from build123d import *

# Parameters (mm, degrees)
F0_R     = 2.5527
F0_R_2   = 14.2875
F0_W     = 25.4
F0_H     = 50.8
F1_DEPTH = 6


with BuildPart() as f1:
    # F0 (on Right) → F1 (new body)
    with BuildSketch(Plane.YZ):
        Polygon((177.8, 139.7), (0, 25.4), (0, -25.4), (177.8, -25.4), (177.8, -139.7), (444.5, -139.7), (444.5, 139.7), align=None)
        with Locations((190.5, -127)):
            Circle(F0_R, mode=Mode.SUBTRACT)
        with Locations((215.9, -127)):
            Circle(F0_R, mode=Mode.SUBTRACT)
        with Locations((190.5, -101.6)):
            Circle(F0_R, mode=Mode.SUBTRACT)
        with Locations((215.9, -101.6)):
            Circle(F0_R, mode=Mode.SUBTRACT)
        with Locations((190.5, -76.2)):
            Circle(F0_R, mode=Mode.SUBTRACT)
        with Locations((215.9, -76.2)):
            Circle(F0_R, mode=Mode.SUBTRACT)
        with Locations((4.77777, -11.90625)):
            Circle(F0_R, mode=Mode.SUBTRACT)
        with Locations((46.02223, -11.90625)):
            Circle(F0_R, mode=Mode.SUBTRACT)
        with Locations((63.5, -12.7)):
            Circle(F0_R, mode=Mode.SUBTRACT)
        with Locations((88.9, -12.7)):
            Circle(F0_R, mode=Mode.SUBTRACT)
        with Locations((190.5, -50.8)):
            Circle(F0_R, mode=Mode.SUBTRACT)
        with Locations((215.9, -50.8)):
            Circle(F0_R, mode=Mode.SUBTRACT)
        with Locations((114.3, -12.7)):
            Circle(F0_R, mode=Mode.SUBTRACT)
        with Locations((139.7, -12.7)):
            Circle(F0_R, mode=Mode.SUBTRACT)
        with Locations((165.1, -12.7)):
            Circle(F0_R, mode=Mode.SUBTRACT)
        with Locations((190.5, -25.4)):
            Circle(F0_R, mode=Mode.SUBTRACT)
        with Locations((215.9, -25.4)):
            Circle(F0_R, mode=Mode.SUBTRACT)
        with Locations((190.5, -12.7)):
            Circle(F0_R, mode=Mode.SUBTRACT)
        with Locations((215.9, -12.7)):
            Circle(F0_R, mode=Mode.SUBTRACT)
        with Locations((241.3, -127)):
            Circle(F0_R, mode=Mode.SUBTRACT)
        with Locations((266.7, -127)):
            Circle(F0_R, mode=Mode.SUBTRACT)
        with Locations((292.1, -127)):
            Circle(F0_R, mode=Mode.SUBTRACT)
        with Locations((317.5, -127)):
            Circle(F0_R, mode=Mode.SUBTRACT)
        with Locations((241.3, -101.6)):
            Circle(F0_R, mode=Mode.SUBTRACT)
        with Locations((266.7, -101.6)):
            Circle(F0_R, mode=Mode.SUBTRACT)
        with Locations((292.1, -101.6)):
            Circle(F0_R, mode=Mode.SUBTRACT)
        with Locations((317.5, -101.6)):
            Circle(F0_R, mode=Mode.SUBTRACT)
        with Locations((342.9, -127)):
            Circle(F0_R, mode=Mode.SUBTRACT)
        with Locations((368.3, -127)):
            Circle(F0_R, mode=Mode.SUBTRACT)
        with Locations((393.7, -127)):
            Circle(F0_R, mode=Mode.SUBTRACT)
        with Locations((419.1, -127)):
            Circle(F0_R, mode=Mode.SUBTRACT)
        with Locations((342.9, -101.6)):
            Circle(F0_R, mode=Mode.SUBTRACT)
        with Locations((368.3, -101.6)):
            Circle(F0_R, mode=Mode.SUBTRACT)
        with Locations((393.7, -101.6)):
            Circle(F0_R, mode=Mode.SUBTRACT)
        with Locations((419.1, -101.6)):
            Circle(F0_R, mode=Mode.SUBTRACT)
        with Locations((25.4, 0)):
            Circle(F0_R_2, mode=Mode.SUBTRACT)
        with Locations((4.77777, 11.90625)):
            Circle(F0_R, mode=Mode.SUBTRACT)
        with Locations((46.02223, 11.90625)):
            Circle(F0_R, mode=Mode.SUBTRACT)
        with Locations((63.5, 12.7)):
            Circle(F0_R, mode=Mode.SUBTRACT)
        with Locations((88.9, 12.7)):
            Circle(F0_R, mode=Mode.SUBTRACT)
        with Locations((114.3, 12.7)):
            Circle(F0_R, mode=Mode.SUBTRACT)
        with Locations((139.7, 12.7)):
            Circle(F0_R, mode=Mode.SUBTRACT)
        with Locations((165.1, 12.7)):
            Circle(F0_R, mode=Mode.SUBTRACT)
        with Locations((190.5, 0)):
            Circle(F0_R, mode=Mode.SUBTRACT)
        with Locations((190.5, 12.7)):
            Circle(F0_R, mode=Mode.SUBTRACT)
        with Locations((215.9, 0)):
            Circle(F0_R, mode=Mode.SUBTRACT)
        with Locations((215.9, 12.7)):
            Circle(F0_R, mode=Mode.SUBTRACT)
        with Locations((190.5, 25.4)):
            Circle(F0_R, mode=Mode.SUBTRACT)
        with Locations((215.9, 25.4)):
            Circle(F0_R, mode=Mode.SUBTRACT)
        with Locations((165.1, 50.8)):
            Rectangle(F0_W, F0_H, mode=Mode.SUBTRACT)
        with Locations((190.5, 50.8)):
            Circle(F0_R, mode=Mode.SUBTRACT)
        with Locations((215.9, 50.8)):
            Circle(F0_R, mode=Mode.SUBTRACT)
        with Locations((190.5, 76.2)):
            Circle(F0_R, mode=Mode.SUBTRACT)
        with Locations((215.9, 76.2)):
            Circle(F0_R, mode=Mode.SUBTRACT)
        with Locations((190.5, 101.6)):
            Circle(F0_R, mode=Mode.SUBTRACT)
        with Locations((215.9, 101.6)):
            Circle(F0_R, mode=Mode.SUBTRACT)
        with Locations((190.5, 127)):
            Circle(F0_R, mode=Mode.SUBTRACT)
        with Locations((215.9, 127)):
            Circle(F0_R, mode=Mode.SUBTRACT)
        with Locations((241.3, 101.6)):
            Circle(F0_R, mode=Mode.SUBTRACT)
        with Locations((266.7, 101.6)):
            Circle(F0_R, mode=Mode.SUBTRACT)
        with Locations((292.1, 101.6)):
            Circle(F0_R, mode=Mode.SUBTRACT)
        with Locations((317.5, 101.6)):
            Circle(F0_R, mode=Mode.SUBTRACT)
        with Locations((241.3, 127)):
            Circle(F0_R, mode=Mode.SUBTRACT)
        with Locations((266.7, 127)):
            Circle(F0_R, mode=Mode.SUBTRACT)
        with Locations((292.1, 127)):
            Circle(F0_R, mode=Mode.SUBTRACT)
        with Locations((317.5, 127)):
            Circle(F0_R, mode=Mode.SUBTRACT)
        with Locations((342.9, 101.6)):
            Circle(F0_R, mode=Mode.SUBTRACT)
        with Locations((368.3, 101.6)):
            Circle(F0_R, mode=Mode.SUBTRACT)
        with Locations((393.7, 101.6)):
            Circle(F0_R, mode=Mode.SUBTRACT)
        with Locations((342.9, 127)):
            Circle(F0_R, mode=Mode.SUBTRACT)
        with Locations((368.3, 127)):
            Circle(F0_R, mode=Mode.SUBTRACT)
        with Locations((419.1, 114.3)):
            Circle(F0_R_2, mode=Mode.SUBTRACT)
        with Locations((393.7, 127)):
            Circle(F0_R, mode=Mode.SUBTRACT)
    extrude(amount=F1_DEPTH)


solid = f1.part
Check sheet for the modelled part. Datum: model origin and axes. Units: mm. Give positions to 0.01 mm unless a question says otherwise; leave off trailing zeros. Write each loop counter-clockwise with the first axis right and the second up, starting at its lowest first coordinate (ties: lowest second). Pieces come first, ordered by that corner, then holes. Notation, with made-up numbers: (-21, 50) -> (-17, 50) arc R32 cw to (-17, 88) -> close; hole circle Ø9 at (13.25, -38). An arc over 180 degrees is marked (long way). Write item = value, one per line.
Item 1: Sectioned sample at B-B on z = -38. Record the boundary of the cut face in (x, y), and give its area (3 significant figures).
Output:
outline = (0, 177.8) -> (6, 177.8) -> (6, 444.5) -> (0, 444.5) -> close
area = 1,600 mm^2
Item 2: Sectioned sample at C-C on x = 1. Count the separate pieces of the cut face and the enclosed holes in it, and give its area (3 significant figures).
Output:
separate_pieces = 1
enclosed_holes = 73
area = 89,700 mm^2
Item 3: Sectioned sample at A-A on y = 25.4. Record the boundary of the cut face in (x, z).
Output:
outline = (0, -25.4) -> (6, -25.4) -> (6, -14.29) -> (0, -14.29) -> close; (0, 14.29) -> (6, 14.29) -> (6, 41.73) -> (0, 41.73) -> close
Item 4: Scan lines: probe 1 along Z at (x, y) = (1, 292); probe 2 along Y at (x, z) = (4.45, 2); probe 3 along Z at (x, y) = (2.45, 47.5). Record each from-to range of solid material in increasing order. Write a range as from..to.
Output:
probe_1 = -139.7..-129.55, -124.45..-104.15, -99.05..99.05, 104.15..124.45, 129.55..139.7
probe_2 = 0..11.25, 39.55..188.91, 192.09..214.31, 217.49..444.5
probe_3 = -25.4..-13.99, -9.82..9.82, 13.99..55.94
Item 5: Sectioned sample at D-D on y = 129. Record the boundary of the cut face in (x, z), and give its area (3 significant figures).
Output:
outline = (0, -25.4) -> (6, -25.4) -> (6, 108.33) -> (0, 108.33) -> close
area = 802 mm^2
Item 6: Gauge pin test, flat ends, axial feed: pin 1 (6.5 mm diameter, centred on y = 215.9, z = 76.2, fed in from -X); pin 2 (1.8 mm diameter, centred on x = 3.5, z = 50, fed in from -Y); pin 3 (1.5 mm diameter, centred on x = 2, z = -88, fed in from -Y). Record the tip position at first contact, or that the pin passes through.
Output:
pin_1 = 0
pin_2 = 36.87
pin_3 = 177.8
Item 7: Release check for a two-part mould opening along Z. For faces 1 (the flat face through (2.958, 90.145, 83.35)), 2 (the flat face through (0, 269, 2)), 3 (the cylindrical face through (2.958, 11.126, 0.628)) record: +Z half, -Z half, draft (parallel to the pull), parting line (faces both ways), or undercut.
Output:
face_1 = +Z half
face_2 = draft
face_3 = undercut
